from build123d import *

# Parameters (mm, degrees)
F1_DEPTH = 25.4


with BuildPart() as f1:
    # F0 (on Front) → F1 (new body)
    with BuildSketch(Plane.XZ):
        with BuildLine():
            Line((-101.154926, 11.54634), (-121.53038, -8.829114))
            Line((-121.53038, -8.829114), (-102.389246, -8.829114))
            ThreePointArc((-102.389246, -8.829114), (11.819616, 7.991988), (126.028478, -8.829114))
            Line((126.028478, -8.829114), (145.16962, -8.829114))
            Line((145.16962, -8.829114), (70.50777, 67.500003))
            Line((70.50777, 67.500003), (-48.560128, 67.500003))
            Line((-48.560128, 67.500003), (-101.154926, 11.54634))
        make_face()
    extrude(amount=F1_DEPTH)


solid = f1.part
For this review, take the finished solid that the model builds, in its own axes (mm). Round coordinates to 2 decimals unless told otherwise and drop trailing zeros. Write each loop counter-clockwise with the first axis right and the second up, starting at its lowest first coordinate (ties: lowest second). Pieces come first, ordered by that corner, then holes. Notation, with made-up numbers: (82, 41.25) - (109, 41.25) arc R4 ccw to (109, 46.25) - close; hole circle Ø10 at (-16, -9.5). An arc over 180 degrees is marked (long way). Write item = value, one per line. Start each with the question number.
1. For pin 1 Ø1.5 at (x, y) = (-32, -8.5) entering from -Z; pin 2 Ø8 at (y, z) = (-11.5, 2) entering from +X; pin 3 Ø1.5 at (x, y) = (-74, -21) entering from +Z, all flat-tipped, find the tip position at first contact; note any pin that passes through.
2. Consider section C-C on x = 17.5. State the section outline as (y, z) points.
3. Wall thickness on L1, parallel to X at y = -12, z = 49; L2, parallel to X at y = -3, z = 43; L3, parallel to Z at x = 73, y = -15.75: over which ranges is each line inside the solid? List them lowest first.
4. Consider section A-A on z = 1. State the section outline as (x, y) points, plus the area to 3 significant figures.
5. Draft analysis for pull direction Y (two halves, no side actions). For faces 1 (the face through (-112, -13, -8.829)), 2 (the face through (10, -25.4, 30)), 3 (the face through (10, 0, 30)), state which applies: released by +Y, released by -Y, zero draft, split by the parting line, or undercut.
6. Consider section B-B on y = -12.25. State the section outline as (x, z) points, plus the area to 3 significant figures.
7. Consider section D-D on z = 43. State the section outline as (x, y) points.
Evaluation:
q1.pin_1 = 5.48
q1.pin_2 = 138.49
q1.pin_3 = 41.23
q2.outline = (-25.4, 7.95) - (0, 7.95) - (0, 67.5) - (-25.4, 67.5) - close
q3.L1 = -65.95 to 88.6
q3.L2 = -71.59 to 94.47
q3.L3 = 3.24 to 64.95
q4.outline = (-111.7, -25.4) - (-62.28, -25.4) - (-62.28, 0) - (-111.7, 0) - close; (85.92, -25.4) - (135.56, -25.4) - (135.56, 0) - (85.92, 0) - close
q4.area = 2,520 mm2
q5.face_1 = zero draft
q5.face_2 = released by -Y
q5.face_3 = released by +Y
q6.outline = (-121.53, -8.83) - (-102.39, -8.83) arc R396.13 cw to (126.03, -8.83) - (145.17, -8.83) - (70.51, 67.5) - (-48.56, 67.5) - (-101.15, 11.55) - close
q6.area = 12,100 mm2
q7.outline = (-71.59, -25.4) - (94.47, -25.4) - (94.47, 0) - (-71.59, 0) - close
